The listing builds one solid part. Answer for the finished solid, in the listing's coordinates (mm). Face numbers are marked on the shaded views. A direction names the side the tool comes from. Coordinates: 2 decimals unless noted, no trailing zeros. Order: outer loops, then holes, each group sorted by start corner. A loop starts at its lowest first (then second) coordinate and runs counter-clockwise, first axis right, second up. Notation, with made-up numbers: (86, 71.5) -> (104, 71.5) arc R17 cw to (104, 95.5) -> close; hole circle Ø9 at (-30, 18.5). An arc over 180 degrees is marked (long way). Put each result on its own line as item: value. Start each with the question number.
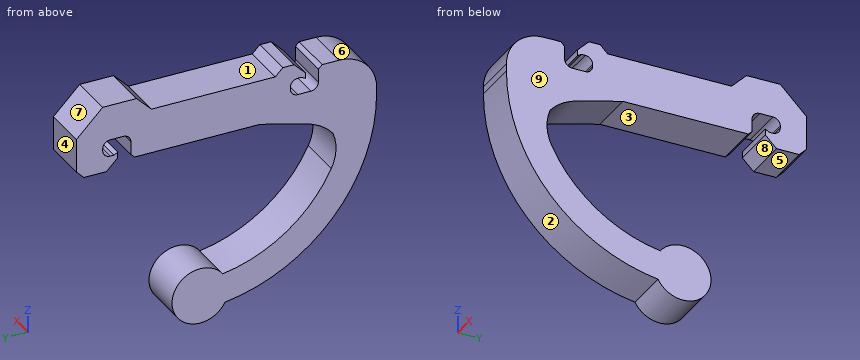
```python
from build123d import *

# Parameters (mm, degrees)
BOSS_EXTRUDE1_DEPTH = 12
FILLET1_R           = 12
FILLET2_R           = 10
CUT_EXTRUDE1_DEPTH  = 12
CHAMFER1_SIZE       = 3
FILLET3_R           = 2
BOSS_EXTRUDE2_DEPTH = 12
BOSS_EXTRUDE3_DEPTH = 12
CHAMFER2_SIZE       = 1


with BuildPart() as part:
    # Sketch2 → Boss-Extrude1 (new body)
    with BuildSketch(Plane(origin=(0, 0, 0), x_dir=(0, 0, -1), z_dir=(1, 0, 0))):
        with BuildLine():
            Line((-6, 40), (6, 40))
            Line((6, 40), (6, -32))
            ThreePointArc((6, -32), (31.376089713, -22.623144998), (44.55766945, 1.001361229))
            ThreePointArc((44.55766945, 1.001361229), (49.578973365, 14.504959969), (52.55766945, 0.409285399))
            ThreePointArc((52.55766945, 0.409285399), (36.824206929, -28.488778663), (6, -40))
            Line((6, -40), (-6, -40))
            Line((-6, -40), (-6, 40))
        make_face()
    extrude(amount=BOSS_EXTRUDE1_DEPTH)

    # Fillet1
    fillet1_edges = [part.edges().sort_by_distance(p)[0] for p in [
        (6, -32, -6),
    ]]
    fillet(fillet1_edges, radius=FILLET1_R)

    # Fillet2
    fillet2_edges = [part.edges().sort_by_distance(p)[0] for p in [
        (6, -40, 6),
    ]]
    fillet(fillet2_edges, radius=FILLET2_R)

    # Sketch3 → Cut-Extrude1 (cut)
    with BuildSketch(Plane(origin=(12, 0, 0), x_dir=(0, 0, -1), z_dir=(1, 0, 0))):
        Polygon((-6, -20), (-4, -20), (-4, -17), (0.5, -17), (0.5, -20), (0.5, -24.5), (-6, -24.5), align=None)
        Polygon((6, 30), (4, 30), (4, 33), (-0.5, 33), (-0.5, 30), (-0.5, 25.5), (6, 25.5), align=None)
    extrude(amount=-CUT_EXTRUDE1_DEPTH, mode=Mode.SUBTRACT)

    # Chamfer1
    chamfer1_edges = [part.edges().sort_by_distance(p)[0] for p in [
        (6, 40, 6),
    ]]
    chamfer(chamfer1_edges, length=CHAMFER1_SIZE)

    # Fillet3
    fillet3_edges = [part.edges().sort_by_distance(p)[0] for p in [
        (6, -17, 4),
        (6, -17, -0.5),
        (6, -24.5, -0.5),
        (6, 25.5, 0.5),
        (6, 33, 0.5),
        (6, 33, -4),
    ]]
    fillet(fillet3_edges, radius=FILLET3_R)

    # Sketch4 → Boss-Extrude2 (add)
    with BuildSketch(Plane(origin=(12, 0, 0), x_dir=(0, 0, -1), z_dir=(1, 0, 0))):
        Polygon((6, 30), (8, 32), (8, 38), (6, 40), align=None)
        Polygon((-6, -20), (-8, -18), (-8, -15), (-6, -13), align=None)
        Polygon((-6, 37), (-10, 33), (-10, 24), (-6, 20), align=None)
        with BuildLine():
            Line((6, -8.96976203), (3.756023672, -12.28945594))
            Line((3.756023672, -12.28945594), (6, -29.586808416))
            Line((6, -29.586808416), (13.733193293, -28.4055347))
            add(Edge.make_bspline(
                [(6, -8.96976203), (8.392195381, -17.703259611), (9.041325817, -20.67605108), (9.22470807, -24.630513259), (13.733193293, -28.4055347)],
                knots=[0, 0, 0, 0, 0, 1, 1, 1, 1, 1], degree=4))
        make_face()
    extrude(amount=-BOSS_EXTRUDE2_DEPTH)

    # Sketch5 → Boss-Extrude3 (add)
    with BuildSketch(Plane(origin=(12, 0, 0), x_dir=(0, 0, -1), z_dir=(1, 0, 0))):
        Polygon((6, 30), (5, 29), (4, 29), (3.422649731, 29), (4, 30), align=None)
        Polygon((-6, -20), (-5, -21), (-4, -21), (-3.422649731, -21), (-4, -20), align=None)
    extrude(amount=-BOSS_EXTRUDE3_DEPTH)

    # Chamfer2
    chamfer2_edges = [part.edges().sort_by_distance(p)[0] for p in [
        (6, -24.5, 6),
        (6, 25.5, -6),
    ]]
    chamfer(chamfer2_edges, length=CHAMFER2_SIZE)


solid = part.part
```
(1) Each of these flat-tipped pins is pushed along its axis until it touches: P1, Ø0.6, axis at x = 4.5, z = 2, coming from the -Y side; P2, Ø0.9, axis at x = 7, y = -16.5, coming from the +Z side; P3, Ø1.3, axis at x = 8, y = -27.5, coming from the +Z side. Where does it stop, or does it pass through?
(2) The part is cut by section C-C on z = -20.5. Determine the outline of the cut face in (x, y), plus the area to 3 significant figures.
(3) The part is cut by section B-B on y = 22.5. Determine the outline of the cut face in (x, z), plus the area to 3 significant figures.
(4) A tool of negligible diameter and unlimited length cuts with its end or side. For the marked faces 1, 2, 3, 4 and 5, from which of +Z, -Z, +X, -X, +Y, -Y can it reach the whole face along a straight path? Write none if from no direction.
(5) The part is cut by section D-D on y = 12. Determine the outline of the cut face in (x, z).
(6) Find the intervals of material crossed by L1, parallel to Z at x = 7.5, y = -18; L2, parallel to Z at x = 7.5, y = 19; L3, parallel to Y at x = 3, z = 0, in increasing order.
(7) The part is cut by section A-A on y = -6. Determine the outline of the cut face in (x, z), plus the area to 3 significant figures.
(8) For a pull along Y with two mould halves and no side action, classify the marked faces 6, 7, 8 and 9 as released by +Y, released by -Y, zero draft, split by the parting line, or undercut.
Worked out:
1. P1: y = -38.22
1. P2: z = 8
1. P3: z = 6
2. outline: (0, -37.71) -> (12, -37.71) -> (12, -28.93) -> (0, -28.93) -> close
2. area: 105 mm2
3. outline: (0, -6) -> (12, -6) -> (12, 8.5) -> (0, 8.5) -> close
3. area: 174 mm2
4. face 1: +Z, +X, -X
4. face 2: -Z, +X, -X, -Y
4. face 3: +X, -X
4. face 4: +Z, -Z, +X, -X, +Y
4. face 5: -Z, +X, -X, +Y
5. outline: (0, -54.64) -> (12, -54.64) -> (12, -43.41) -> (0, -43.41) -> close; (0, -6) -> (12, -6) -> (12, 6) -> (0, 6) -> close
6. L1: -45.81 to -35.95, -8.34 to -0.23, 3.73 to 8
6. L2: -6 to 6
6. L3: -39.17 to -23.82, -17.68 to 26.18, 32.32 to 40
7. outline: (0, -51.19) -> (12, -51.19) -> (12, -42.79) -> (0, -42.79) -> close; (0, -6) -> (12, -6) -> (12, 6) -> (0, 6) -> close
7. area: 245 mm2
8. face 6: released by -Y
8. face 7: released by +Y
8. face 8: undercut
8. face 9: zero draft
